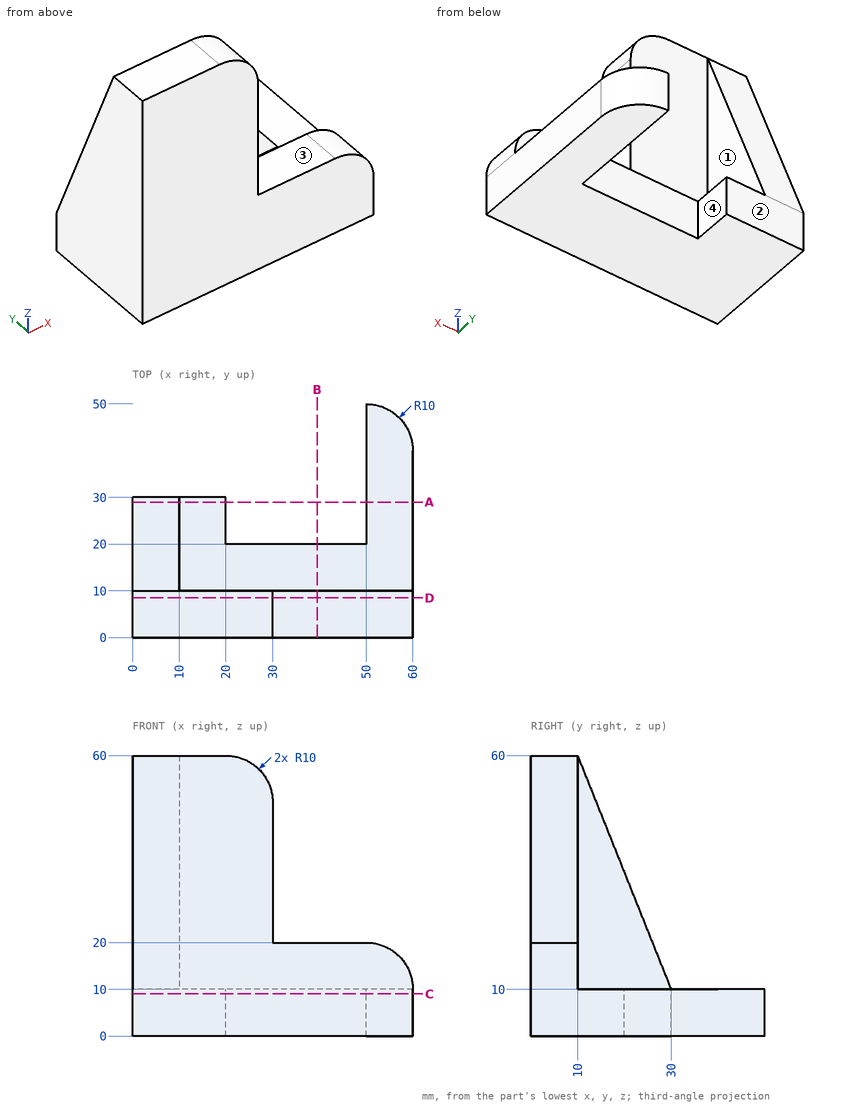
Study the drawing (mm; zero at the part's minimum x, y, z) and answer. A direction names the side the tool comes from. Round coordinates to 2 decimals unless told otherwise and drop trailing zeros. Order: outer loops, then holes, each group sorted by start corner. A loop starts at its lowest first (then second) coordinate and runs counter-clockwise, first axis right, second up. Notation, with made-up numbers: (-36.5, 34.5) - (2.5, 34.5) arc R17 ccw to (2.5, 40.5) - close; hole circle Ø11 at (45.25, 29.5). An arc over 180 degrees is marked (long way). Use one line per item in the form item = value. Start each with the question number.
(1) Flat-ended cylindrical pins translate along their axes: pin 1 Ø11 at (x, z) = (39.5, 3) entering from +Y; pin 2 Ø8 at (y, z) = (35, 4.5) entering from -X; pin 3 Ø8 at (x, y) = (39.5, 4.5) entering from +Z; pin 4 Ø5 at (x, y) = (29.5, 13) entering from -Z. Find the tip coordinate at first contact, or state that the pin passes through.
(2) The part is cut by section D-D (y = 8.5). Give the vertices of the cut face in (x, z), then the cut area to 3 significant figures.
(3) For the marked faces 1, 2, 3 and 4, determine the directions among +Z, -Z, +X, -X, +Y, -Y from which every point of the face is accessible in a straight line to the end or side of a thin tool.
(4) The part is cut by section A-A (y = 29). Give the vertices of the cut face in (x, z).
(5) The part is cut by section C-C (z = 9). Give the vertices of the cut face in (x, y).
(6) Find the intervals of material crossed by line 1 along X through (y, z) = (25, 8); line 2 along Z through (x, y) = (52.5, 25); line 3 along X through (y, z) = (35, 8), in increasing order. Write a range as from..to.
(7) The part is cut by section B-B (x = 39.5). Give the vertices of the cut face in (y, z), then the cut area to 3 significant figures.
Checked values:
q1.pin_1 = 20
q1.pin_2 = 50
q1.pin_3 = 20
q1.pin_4 = 0
q2.outline = (0, 0) - (60, 0) - (60, 10) arc R10 ccw to (50, 20) - (30, 20) - (30, 50) arc R10 ccw to (20, 60) - (0, 60) - close
q2.area = 2,360 mm^2
q3.face_1 = +Z, +X, +Y
q3.face_2 = +Z, -Z, -X, +Y
q3.face_3 = +Z, +X, +Y, -Y
q3.face_4 = +Z, -Z, +Y
q4.outline = (0, 0) - (20, 0) - (20, 10) - (10, 10) - (10, 12.5) - (0, 12.5) - close; (50, 0) - (60, 0) - (60, 10) - (50, 10) - close
q5.outline = (0, 0) - (60, 0) - (60, 40) arc R10 ccw to (50, 50) - (50, 20) - (20, 20) - (20, 30) - (0, 30) - close
q6.line_1 = 0..20, 50..60
q6.line_2 = 0..10
q6.line_3 = 50..60
q7.outline = (0, 0) - (20, 0) - (20, 10) - (10, 10) - (10, 20) - (0, 20) - close
q7.area = 300 mm^2
